Check sheet for the modelled part. Datum: model origin and axes. Units: mm. A direction names the side the tool comes from. Give positions to 0.01 mm unless a question says otherwise; leave off trailing zeros. Loops run counter-clockwise (first coordinate to the right, second up) from the corner with the lowest first, then second, coordinate; pieces in that order, holes last. Notation, with made-up numbers: (46.25, 26) - (53.25, 26) arc R21 ccw to (53.25, 55) - close; hole circle Ø9 at (24, 42.5). An arc over 180 degrees is marked (long way). Answer in a Markdown table with one row per item. Add a question column.
(1) Sectioned sample at A-A on x = 3. Enter the section's corners in (y, z), then the cut area to 3 significant figures.
(2) Sectioned sample at C-C on x = 7. Enter the section's corners in (y, z).
(3) Thickness scan on L1, parallel to Z at x = -5.5, y = 6; L2, parallel to X at y = 1.5, z = 53; L3, parallel to X at y = 1, z = 57. Record the ranges inside material, lowest first.
(4) Sectioned sample at B-B on y = 7.25. Enter the section's corners in (x, z), then the cut area to 3 significant figures.
(5) Sectioned sample at D-D on y = 3. Enter the section's corners in (x, z).
(6) Set-up check for faces 4 (the face through (1.08, -4.88, 46.49)), 5 (the face through (0, 8.227, 90)): record each of +Z, -Z, +X, -X, +Y, -Y from which the full face is reachable in a straight line by a thin tool's end or side.
(7) Go/stop test with flat-tipped pins: P1, Ø2, axis at x = -0.5, z = 31, coming from the +Y side; P2, Ø6, axis at y = -2.5, z = 67.5, coming from the -X side; P3, Ø5, axis at x = -0.5, z = 71, coming from the -Y side; P4, Ø1, axis at x = -6.5, z = 35.5, coming from the -Y side. Record where each tip stops, or that it passes through.
(8) Draft check along Z on faces 1 (the face through (0, 0, 94.044)), 2 (the face through (4, 4, 8.89)), 3 (the face through (7.158, -4.056, 4.383)). Enter one of: released by +Z, released by -Z, zero draft, split by the parting line, or undercut.
Autodesk Inventor part; units mm, degrees
ref_plane "YZ Plane" through (0, 0, 0) normal (1, 0, 0) x (0, 1, 0)
ref_plane "XZ Plane" through (0, 0, 0) normal (0, 1, 0) x (-1, 0, 0)
ref_plane "XY Plane" through (0, 0, 0) normal (0, 0, 1) x (1, 0, 0)
sketch "Sketch1" plane through (0, 0, 0) normal (0, 0, 1) x (1, 0, 0)
  circle A0 centre (0, 0) radius 5
  circle A1 centre (0, 0) radius 9.5
  line L0 (-4.75, 8.2272) -> (4.75, 8.2272)
  line L1 (4.75, 8.2272) -> (9.5, 0)
  line L2 (9.5, 0) -> (4.75, -8.2272)
  line L3 (4.75, -8.2272) -> (-4.75, -8.2272)
  line L4 (-4.75, -8.2272) -> (-9.5, 0)
  line L5 (-9.5, 0) -> (-4.75, 8.2272)
  dimension "d0" = 10
  dimension "d1" = 19
extrude "Extrusion1" add sketch "Sketch1" along normal blind 8.89 contours L2 L3 L4 L5 L0 L1
sketch "Sketch2" plane through (0, 0, 0) normal (0, 0, -1) x (-1, 0, 0)
  circle A0 centre (0, 0) radius 5
  dimension "d4" = 10
extrude "Extrusion2" add sketch "Sketch2" against normal blind 94.0435
sketch "Sketch3" plane through (0, 0, 94.0435) normal (0, 0, 1) x (1, 0, 0)
  line L0 (-4.75, 8.2272) -> (-9.5, 0)
  circle A0 centre (0, 0) radius 9.5
  line L1 (-9.5, 0) -> (-4.75, 8.2272)
  line L2 (4.75, 8.2272) -> (-4.75, 8.2272)
  line L3 (-4.75, 8.2272) -> (4.75, 8.2272)
  line L4 (9.5, 0) -> (4.75, 8.2272)
  line L5 (4.75, 8.2272) -> (9.5, 0)
  line L6 (9.5, 0) -> (4.75, -8.2272)
  line L7 (4.75, -8.2272) -> (-4.75, -8.2272)
  line L8 (-4.75, -8.2272) -> (-9.5, 0)
extrude "Extrusion3" add sketch "Sketch3" against normal blind 8.89 contours L2 L4 L6 L7 L8 L0
properties part number "hing rod"
Reply:
| question | item | result |
|---|---|---|
| 1 | outline | (-8.23, 0) - (8.23, 0) - (8.23, 8.89) - (4, 8.89) - (4, 85.15) - (8.23, 85.15) - (8.23, 94.04) - (-8.23, 94.04) - (-8.23, 85.15) - (-4, 85.15) - (-4, 8.89) - (-8.23, 8.89) - close |
| 1 | area | 903 mm^2 |
| 2 | outline | (-4.33, 0) - (4.33, 0) - (4.33, 8.89) - (-4.33, 8.89) - close; (-4.33, 85.15) - (4.33, 85.15) - (4.33, 94.04) - (-4.33, 94.04) - close |
| 3 | L1 | 0 to 8.89, 85.15 to 94.04 |
| 3 | L2 | -4.77 to 4.77 |
| 3 | L3 | -4.9 to 4.9 |
| 4 | outline | (-5.31, 0) - (5.31, 0) - (5.31, 8.89) - (-5.31, 8.89) - close; (-5.31, 85.15) - (5.31, 85.15) - (5.31, 94.04) - (-5.31, 94.04) - close |
| 4 | area | 189 mm^2 |
| 5 | outline | (-7.77, 0) - (7.77, 0) - (7.77, 8.89) - (4, 8.89) - (4, 85.15) - (7.77, 85.15) - (7.77, 94.04) - (-7.77, 94.04) - (-7.77, 85.15) - (-4, 85.15) - (-4, 8.89) - (-7.77, 8.89) - close |
| 6 | face 4 | none |
| 6 | face 5 | +Z, -Z, +X, -X, +Y |
| 7 | P1 | y = 5 |
| 7 | P2 | x = -5 |
| 7 | P3 | y = -5 |
| 7 | P4 | through |
| 8 | face 1 | released by +Z |
| 8 | face 2 | undercut |
| 8 | face 3 | zero draft |
